Geometry check sheet. Reference: drawing and pictorial views, mm from the part's lowest x, y, z. Round coordinates to 2 decimals unless told otherwise and drop trailing zeros. Write each loop counter-clockwise with the first axis right and the second up, starting at its lowest first coordinate (ties: lowest second). Pieces come first, ordered by that corner, then holes. Notation, with made-up numbers: M 69.25,50 L 91.25,50 A34 ccw 91.25,84 Z; hole C -29.5,48 d11. An arc over 180 degrees is marked long. Answer in a Markdown table with one row per item.
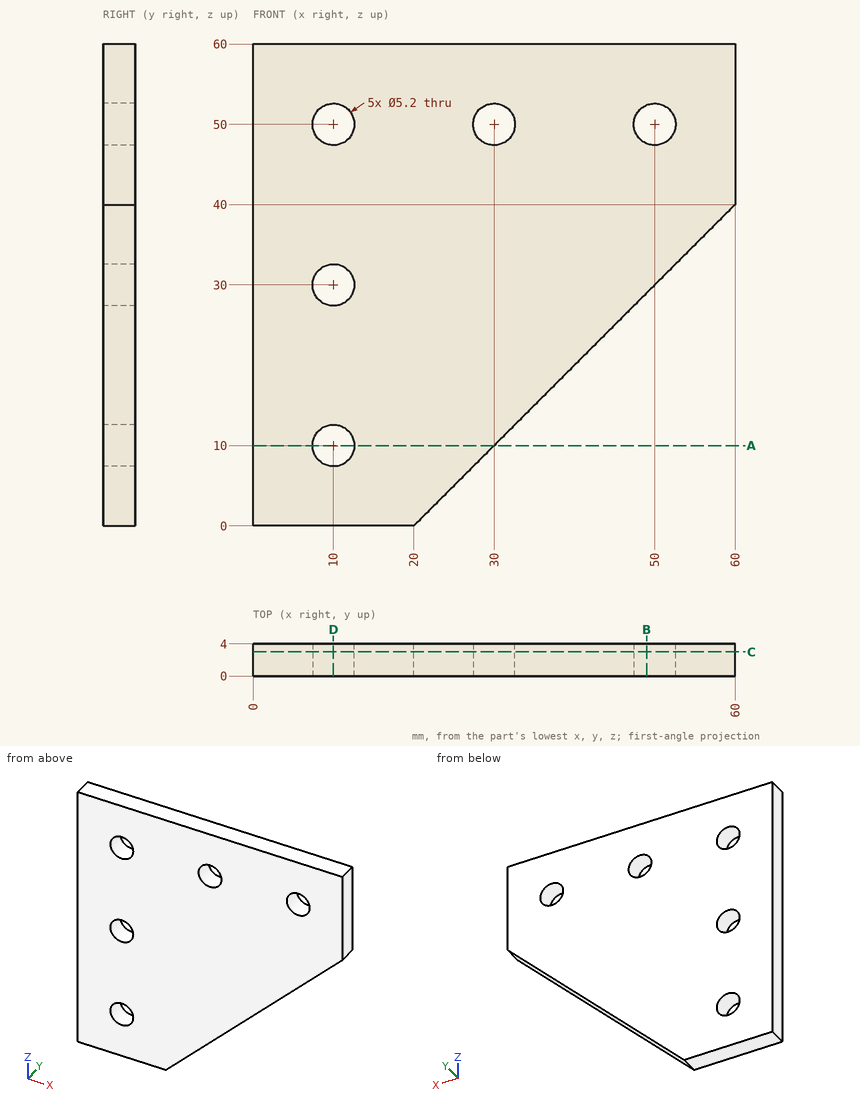
1. Scan lines: L1, parallel to Z at x = 10, y = 1.8; L2, parallel to X at y = 0.4, z = 48.5; L3, parallel to Z at x = 24, y = 1.5. Record each from-to range of solid material in increasing order.
Found:
| item | result |
|---|---|
| L1 | z = 0 to 7.4, 12.6 to 27.4, 32.6 to 47.4, 52.6 to 60 |
| L2 | x = 0 to 7.88, 12.12 to 27.88, 32.12 to 47.88, 52.12 to 60 |
| L3 | z = 4 to 60 |
2. Section check B-B, the plane x = 49. Record the cut outline in (y, z), and give its area (3 significant figures).
Found:
| item | result |
|---|---|
| outline | M 0,29 L 4,29 L 4,47.6 L 0,47.6 Z; M 0,52.4 L 4,52.4 L 4,60 L 0,60 Z |
| area | 105 mm2 |
3. Section check D-D, the plane x = 10. Record the cut outline in (y, z), and give its area (3 significant figures).
Found:
| item | result |
|---|---|
| outline | M 0,0 L 4,0 L 4,7.4 L 0,7.4 Z; M 0,12.6 L 4,12.6 L 4,27.4 L 0,27.4 Z; M 0,32.6 L 4,32.6 L 4,47.4 L 0,47.4 Z; M 0,52.6 L 4,52.6 L 4,60 L 0,60 Z |
| area | 178 mm2 |
4. Go/stop test with a flat-tipped pin: pin 1 (3 mm diameter, centred on x = 50, z = 50, fed in from -Y). Record where the tip stops, or that it passes through.
Found:
| item | result |
|---|---|
| pin 1 | passes through |
5. Section check C-C, the plane y = 3. Record the cut outline in (x, z).
Found:
| item | result |
|---|---|
| outline | M 0,0 L 20,0 L 60,40 L 60,60 L 0,60 Z; hole C 10,10 d5.2; hole C 10,30 d5.2; hole C 10,50 d5.2; hole C 30,50 d5.2; hole C 50,50 d5.2 |
6. Section check A-A, the plane z = 10. Record the cut outline in (x, y).
Found:
| item | result |
|---|---|
| outline | M 0,0 L 7.4,0 L 7.4,4 L 0,4 Z; M 12.6,0 L 30,0 L 30,4 L 12.6,4 Z |
